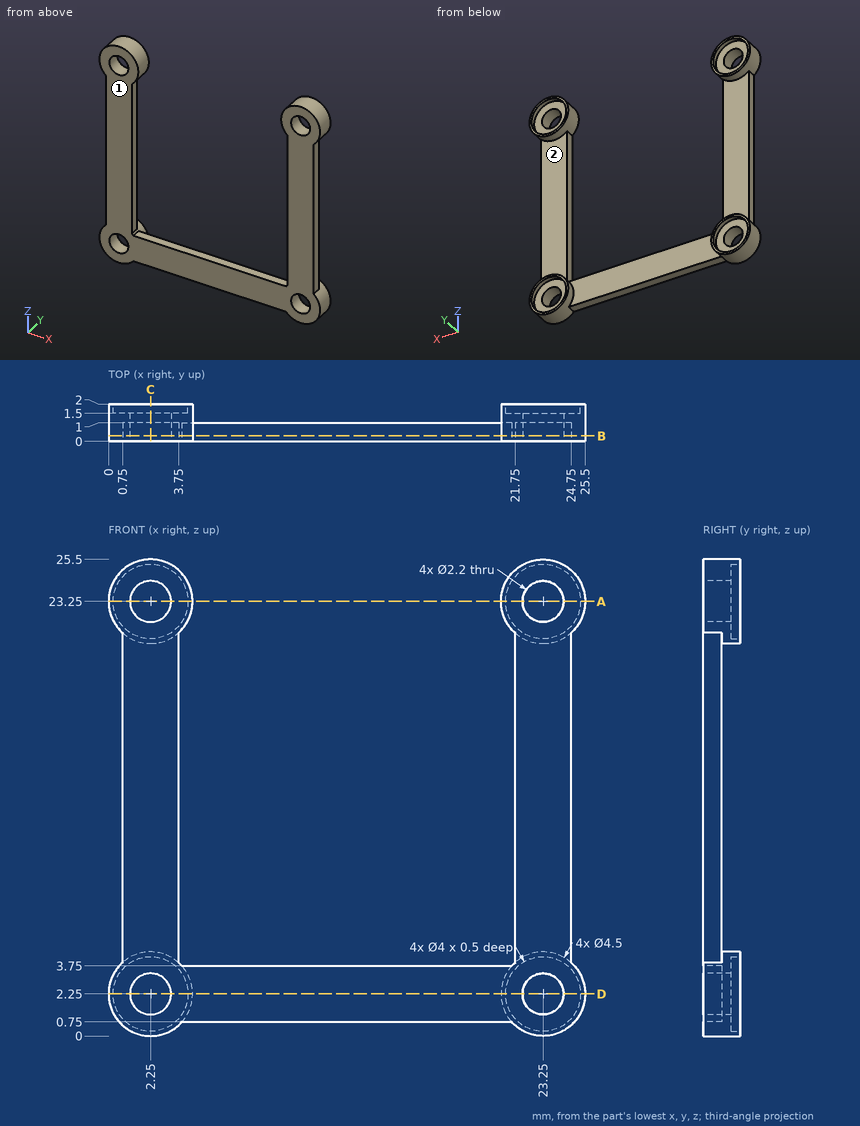
Design review of the part shown in the three views and the two pictorial views. Dimensions are in mm from the part's minimum x, y and z. Coordinates: 2 decimals unless noted, no trailing zeros. Write each loop counter-clockwise with the first axis right and the second up, starting at its lowest first coordinate (ties: lowest second). Pieces come first, ordered by that corner, then holes.
(1) Add section A-A on z = 23.25. Give the boundary of the cut face in (x, y), then the cut area to 3 significant figures.
(2) Wall thickness on probe 1 along Z at (x, y) = (2.25, 1.75); probe 2 along Z at (x, y) = (23.25, 0.45); probe 3 along X at (y, z) = (1, 23.25): over which ranges is each line inside the solid? List them lowest first.
(3) Add section B-B on y = 0.3. Give the boundary of the cut face in (x, z).
(4) Add section D-D on z = 2.25. Give the boundary of the cut face in (x, y), then the cut area to 3 significant figures.
(5) For pin 1 Ø0.8 at (y, z) = (0.5, 12) entering from -X; pin 2 Ø2.5 at (x, z) = (14.5, 1.5) entering from +Y; pin 3 Ø2 at (x, z) = (2.25, 23.25) entering from -Y; pin 4 Ø1.1 at (y, z) = (0.5, 16.5) entering from +X, all flat-tipped, find the tip position at first contact; note any pin that passes through.
(6) Add section C-C on x = 2.25. Give the boundary of the cut face in (y, z).
(7) The part is to be moulded in two halves that separate along Z. For the marked faces 1 and 2, say which applies: +Z half, -Z half, draft (parallel to the pull), parting line (faces both ways), or undercut.
Answer sheet:
1. outline: (0, 0) - (1.15, 0) - (1.15, 1.5) - (0.25, 1.5) - (0.25, 2) - (0, 2) - close; (3.35, 0) - (4.5, 0) - (4.5, 2) - (4.25, 2) - (4.25, 1.5) - (3.35, 1.5) - close; (21, 0) - (22.15, 0) - (22.15, 1.5) - (21.25, 1.5) - (21.25, 2) - (21, 2) - close; (24.35, 0) - (25.5, 0) - (25.5, 2) - (25.25, 2) - (25.25, 1.5) - (24.35, 1.5) - close
1. area: 7.40 mm2
2. probe 1: z = 0 to 0.25, 4.25 to 4.5, 21 to 21.25, 25.25 to 25.5
2. probe 2: z = 0 to 1.15, 3.35 to 22.15, 24.35 to 25.5
2. probe 3: x = 0 to 1.15, 3.35 to 4.5, 21 to 22.15, 24.35 to 25.5
3. outline: (0.75, 3.93) arc R2.25 ccw (long way) to (3.93, 0.75) - (21.57, 0.75) arc R2.25 ccw (long way) to (24.75, 3.93) - (24.75, 21.57) arc R2.25 ccw (long way) to (21.75, 21.57) - (21.75, 3.93) arc R2.25 ccw to (21.57, 3.75) - (3.93, 3.75) arc R2.25 ccw to (3.75, 3.93) - (3.75, 21.57) arc R2.25 ccw (long way) to (0.75, 21.57) - close; hole circle Ø2.2 at (2.25, 2.25); hole circle Ø2.2 at (2.25, 23.25); hole circle Ø2.2 at (23.25, 2.25); hole circle Ø2.2 at (23.25, 23.25)
4. outline: (0, 0) - (1.15, 0) - (1.15, 1.5) - (0.25, 1.5) - (0.25, 2) - (0, 2) - close; (3.35, 0) - (22.15, 0) - (22.15, 1.5) - (21.25, 1.5) - (21.25, 2) - (21, 2) - (21, 1) - (4.5, 1) - (4.5, 2) - (4.25, 2) - (4.25, 1.5) - (3.35, 1.5) - close; (24.35, 0) - (25.5, 0) - (25.5, 2) - (25.25, 2) - (25.25, 1.5) - (24.35, 1.5) - close
4. area: 23.9 mm2
5. pin 1: stops at x = 0.75
5. pin 2: stops at y = 1
5. pin 3: passes through
5. pin 4: stops at x = 24.75
6. outline: (0, 0) - (2, 0) - (2, 0.25) - (1.5, 0.25) - (1.5, 1.15) - (0, 1.15) - close; (0, 3.35) - (1.5, 3.35) - (1.5, 4.25) - (2, 4.25) - (2, 4.5) - (1, 4.5) - (1, 21) - (2, 21) - (2, 21.25) - (1.5, 21.25) - (1.5, 22.15) - (0, 22.15) - close; (0, 24.35) - (1.5, 24.35) - (1.5, 25.25) - (2, 25.25) - (2, 25.5) - (0, 25.5) - close
7. face 1: draft
7. face 2: undercut
